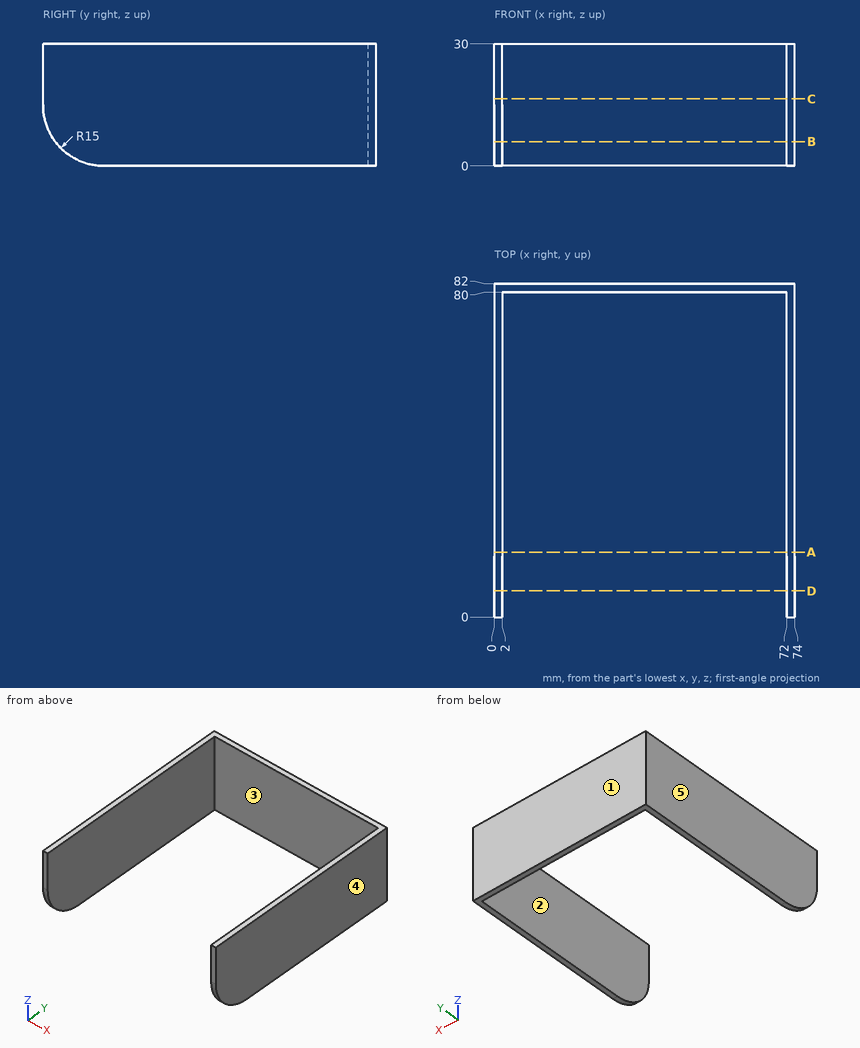
Study the drawing (mm; zero at the part's minimum x, y, z) and answer. A direction names the side the tool comes from. Give positions to 0.01 mm unless a question says otherwise; leave off trailing zeros. Loops run counter-clockwise (first coordinate to the right, second up) from the corner with the lowest first, then second, coordinate; pieces in that order, holes last. Notation, with made-up numbers: (29, 11) -> (85, 11) arc R27 cw to (85, 47) -> close; hole circle Ø3 at (-10.75, -2). An arc over 180 degrees is marked (long way). Write item = value, one per line. Start each with the question number.
(1) Which of the six approach directions +Z, -Z, +X, -X, +Y, -Y give full straight-line access (tool end or side, diameter ignored) to the marked faces 1 and 2?
(2) The mould has two halves that part along X. Classify the marked faces 3, 4 and 5: +X half, -X half, draft (parallel to the pull), parting line (faces both ways), or undercut.
(3) Find section B-B on z = 6. Give the vertices of the cut face in (x, y), and give its area (3 significant figures).
(4) Find section C-C on z = 16.5. Give the vertices of the cut face in (x, y).
(5) Given pin 1 Ø15 at (y, z) = (45.5, 12.5) entering from -X; pin 2 Ø4 at (x, z) = (29, 20) entering from -Y, each flat-ended and moving along its own axis, determine where each tip first touches the part or whether it passes through.
(6) Find section A-A on y = 16. Give the vertices of the cut face in (x, z).
(7) Find the intervals of material crossed by probe 1 along X at (y, z) = (54, 4.75); probe 2 along Y at (x, z) = (57, 2.5), in increasing order. Write a range as from..to.
(8) Find section D-D on y = 6.5. Give the vertices of the cut face in (x, z).
From the geometry:
q1.face_1 = +Z, -Z, +X, -X, +Y
q1.face_2 = +Z, -Z, -Y
q2.face_3 = undercut
q2.face_4 = +X half
q2.face_5 = -X half
q3.outline = (0, 3) -> (2, 3) -> (2, 80) -> (72, 80) -> (72, 3) -> (74, 3) -> (74, 82) -> (0, 82) -> close
q3.area = 456 mm^2
q4.outline = (0, 0) -> (2, 0) -> (2, 80) -> (72, 80) -> (72, 0) -> (74, 0) -> (74, 82) -> (0, 82) -> close
q5.pin_1 = 0
q5.pin_2 = 80
q6.outline = (0, 0) -> (2, 0) -> (2, 30) -> (0, 30) -> close; (72, 0) -> (74, 0) -> (74, 30) -> (72, 30) -> close
q7.probe_1 = 0..2, 72..74
q7.probe_2 = 80..82
q8.outline = (0, 2.64) -> (2, 2.64) -> (2, 30) -> (0, 30) -> close; (72, 2.64) -> (74, 2.64) -> (74, 30) -> (72, 30) -> close
